Geometry: final body of the model. Coordinates: model frame, mm. A direction names the side the tool comes from. Give positions to 0.01 mm unless a question says otherwise; leave off trailing zeros. Write each loop counter-clockwise with the first axis right and the second up, starting at its lowest first coordinate (ties: lowest second). Pieces come first, ordered by that corner, then holes.
Q1. Line query: line 1 (Y direction, x = 40, z = 53); line 2 (X direction, y = -10, z = 58); line 3 (Z direction, x = -63.5, y = -18.5). Output: solid intervals per line, ascending.
Q2. Section C-C (z = 27). Return the cut outline in (x, y), plus the area to 3 significant figures.
Q3. Mould query, pull axis X, two halves, no side actions, for faces 1 (the flat face through (-1, -30, 30)), 2 (the cylindrical face through (68, -29, 30)), 3 (the flat face through (40, 0, 50)). Classes: +X half, -X half, draft (parallel to the pull), parting line (faces both ways), or undercut.
Q4. Pin query (flat end, axial travel): pin 1 Ø16 at (x, y) = (39.5, -3.5) entering from +Z; pin 2 Ø5 at (x, y) = (6, -6.5) entering from +Z; pin 3 Ø5 at (x, y) = (-50.5, -18.5) entering from +Z. Return the tip coordinate at first contact, or that it passes through.
Q5. Section A-A (y = 0). Return the cut outline in (x, z).
Q6. Section B-B (x = 0). Return the cut outline in (y, z), plus the area to 3 significant figures.
Q7. Section D-D (x = -19). Return the cut outline in (y, z).
Q8. Reachability of faces 4 (the cylindrical face through (-50, 0, 67)), 5 (the cylindrical face through (68, 29, 30)) from +Z, -Z, +X, -X, +Y, -Y: full face, straight path, thin tool, end or side. Return the list, or none.
from build123d import *

# Parameters (mm, degrees)
F0_W     = 140
F0_H     = 60
F1_DEPTH = 60
F2_R     = 10
F5_DEPTH = 10
F3_R     = 10
F6_DEPTH = 10
F4_R     = 10
F7_DEPTH = 132.8
F8_R     = 5


with BuildPart() as f1:
    # F0 (on Top) → F1 (new body)
    with BuildSketch(Plane.XY):
        Rectangle(F0_W, F0_H)
    extrude(amount=F1_DEPTH)

    # F2 (on face) → F5 (join)
    with BuildSketch(Plane.XY.offset(60)):
        with Locations((-40, 0)):
            Circle(F2_R)
    extrude(amount=F5_DEPTH)

    # F3 (on face) → F6 (cut)
    with BuildSketch(Plane.XY.offset(60)):
        with Locations((40, 0)):
            Circle(F3_R)
    extrude(amount=-F6_DEPTH, mode=Mode.SUBTRACT)

    # F4 (on face) → F7 (cut)
    with BuildSketch(Plane.XY.offset(60)):
        Circle(F4_R)
    extrude(amount=-F7_DEPTH, mode=Mode.SUBTRACT)

    # F8
    f8_edges = [f1.edges().sort_by_distance(p)[0] for p in [
        (-70, 0, 60),
        (0, 30, 60),
        (0, -30, 60),
        (70, 0, 60),
        (-50, 0, 60),
        (-10, 0, 60),
        (30, 0, 60),
        (0, 30, 0),
        (-70, 30, 30),
        (70, 30, 30),
        (-70, -30, 30),
        (-70, 0, 0),
        (0, -30, 0),
        (-10, 0, 0),
        (70, 0, 0),
        (70, -30, 30),
    ]]
    fillet(f8_edges, radius=F8_R)


solid = f1.part
Computed:
1. line 1: y = -30 to -10, 10 to 30
1. line 2: x = -69 to -4.58, 4.58 to 35.42, 44.58 to 69
1. line 3: z = 0 to 60
2. outline: (-70, -25) arc R5 ccw to (-65, -30) - (65, -30) arc R5 ccw to (70, -25) - (70, 25) arc R5 ccw to (65, 30) - (-65, 30) arc R5 ccw to (-70, 25) - close; hole circle Ø20 at (0, 0)
2. area: 8,060 mm2
3. face 1: draft
3. face 2: +X half
3. face 3: undercut
4. pin 1: stops at z = 58.61
4. pin 2: stops at z = 58.41
4. pin 3: stops at z = 60
5. outline: (-70, 5) arc R5 ccw to (-65, 0) - (-15, 0) arc R5 ccw to (-10, 5) - (-10, 55) arc R5 ccw to (-15, 60) - (-25, 60) arc R5 cw to (-30, 65) - (-30, 70) - (-50, 70) - (-50, 65) arc R5 cw to (-55, 60) - (-65, 60) arc R5 ccw to (-70, 55) - close; (10, 5) arc R5 ccw to (15, 0) - (65, 0) arc R5 ccw to (70, 5) - (70, 55) arc R5 ccw to (65, 60) - (55, 60) arc R5 ccw to (50, 55) - (50, 50) - (30, 50) - (30, 55) arc R5 ccw to (25, 60) - (15, 60) arc R5 ccw to (10, 55) - close
6. outline: (-30, 5) arc R5 ccw to (-25, 0) - (-15, 0) arc R5 ccw to (-10, 5) - (-10, 55) arc R5 ccw to (-15, 60) - (-25, 60) arc R5 ccw to (-30, 55) - close; (10, 5) arc R5 ccw to (15, 0) - (25, 0) arc R5 ccw to (30, 5) - (30, 55) arc R5 ccw to (25, 60) - (15, 60) arc R5 ccw to (10, 55) - close
6. area: 2,360 mm2
7. outline: (-30, 5) arc R5 ccw to (-25, 0) - (25, 0) arc R5 ccw to (30, 5) - (30, 55) arc R5 ccw to (25, 60) - (-25, 60) arc R5 ccw to (-30, 55) - close
8. face 4: +Z
8. face 5: +Z, -Z, +X, +Y
